Autodesk Inventor part; units mm, degrees
ref_plane "YZ Plane" through (0, 0, 0) normal (1, 0, 0) x (0, 1, 0)
ref_plane "XZ Plane" through (0, 0, 0) normal (0, 1, 0) x (-1, 0, 0)
ref_plane "XY Plane" through (0, 0, 0) normal (0, 0, 1) x (1, 0, 0)
sketch "Sketch1" plane through (0, 0, 0) normal (1, 0, 0) x (0, 1, 0)
  line L0 (-219.6367, 33.4515) -> (-197.6397, 20.7515)
  line L1 (-197.6397, 20.7515) -> (-184.9397, 42.7485)
  line L2 (-184.9397, 42.7485) -> (-206.9367, 55.4485)
  line L3 (-206.9367, 55.4485) -> (-219.6367, 33.4515)
  line L4 (-219.6367, 33.4515) -> (-184.9397, 42.7485) construction
  line L5 (-197.6397, 20.7515) -> (-206.9367, 55.4485) construction
  circle A0 centre (-38.1, 41.275) radius 38.1
  line L6 (0, 0) -> (-228.6, 0)
  line L7 (-228.6, 0) -> (-228.6, -25.4)
  line L8 (-228.6, -25.4) -> (0, -25.4)
  line L9 (0, -25.4) -> (0, 0)
  line L10 (0, 0) -> (-228.6, -25.4) construction
  line L11 (-228.6, 0) -> (0, -25.4) construction
  line L12 (-38.1, 3.175) -> (-132.0434, 3.175)
  arc A1 (-197.6397, 20.7515) -> (-132.0434, 3.175) centre (-132.0434, 134.3676) ccw
  circle A2 centre (-38.1, 41.275) radius 44.45
  arc A3 (-184.9397, 42.7485) -> (-79.7897, 25.8552) centre (-110.2136, 172.1778) ccw
  circle A4 centre (-101.6, 41.275) radius 7.3323
  line L13 (-107.95, 44.9412) -> (-101.6, 48.6073)
  line L14 (-101.6, 48.6073) -> (-95.25, 44.9412)
  line L15 (-95.25, 44.9412) -> (-95.25, 37.6088)
  line L16 (-95.25, 37.6088) -> (-101.6, 33.9427)
  line L17 (-101.6, 33.9427) -> (-107.95, 37.6088)
  line L18 (-107.95, 37.6088) -> (-107.95, 44.9412)
  point P0 (-202.2882, 38.1)
  point P1 (-114.3, -12.7)
  point P2 (-60.9953, 3.175)
  dimension "d0" = 76.2
  dimension "d1" = 25.4
  dimension "d2" = 60
  dimension "d3" = 41.275
  dimension "d4" = 38.1
  dimension "d5" = 146.847
  dimension "d6" = 20.7515
  dimension "d7" = 228.6
  dimension "d8" = 88.9
  dimension "d23" = 12.7
  dimension "d24" = 63.5
extrude "Extrusion1" add sketch "Sketch1" along normal mid plane 177.8 contours L1 A3 A2 L12 A1
sketch "Sketch2" plane through (-88.9, -197.6397, 20.7515) normal (0, -0.866, 0.5) x (1, 0, 0)
  line L0 (0, 0) -> (177.8, 0)
  line L1 (177.8, 25.4) -> (177.8, 0)
  point P0 (88.9, 80.8485)
  point P1 (152.4, 12.7)
  dimension "d11" = 12.7
  dimension "d12" = 25.4
hole "Hole1" at (63.5, -191.2897, 31.75) direction (0, 0.866, -0.5) diameter 4.445 depth 38.1 counterbore diameter 5.588 counterbore depth 8.255
pattern_linear "Rectangular Pattern1" count 6 spacing 25.4 along (-1, 0, 0) of "Hole1"
properties part number "FlyWheel Alligner"
Part model, mm, in its own coordinate system. A direction names the side the tool comes from. Give positions to 0.01 mm unless a question says otherwise; leave off trailing zeros. Write each loop counter-clockwise with the first axis right and the second up, starting at its lowest first coordinate (ties: lowest second). Pieces come first, ordered by that corner, then holes. Notation, with made-up numbers: (77.25, -20) -> (128.25, -20) arc R22 ccw to (128.25, 14) -> close; hole circle Ø11 at (-18.75, 79). An arc over 180 degrees is marked (long way). Put each result on its own line as item: value. Start each with the question number.
Item 1: Which spindle directions (+Z, -Z, +X, -X, +Y, -Y) get a long thin tool onto all of the face, cutting with end or side? Do faces 4 (the face through (-1.24, -133.17, 24.5)), 5 (the face through (-38.131, -158.279, 12.727)). Say none if no direction does.
Item 2: Cut at B-B (y = -113.5). List the corners of the cut face in (x, z) (3 decimals), then the cut area to 3 significant figures.
Item 3: Pull direction X, two halves, no side cores. Call faces 1 (the face through (-35.62, -188.31, 28.54)), 2 (the face through (-1, -96, 3.175)), 3 (the face through (-88.9, -130, 19)): pulls with the +X half, pulls with the -X half, needs draft (parallel to the pull), parting line crosses it, or undercut.
Item 4: Cut at C-C (z = 36.5). List the corners of the cut face in (x, y), then the cut area to 3 significant figures.
Item 5: Pin check, flat tips, straight feed: pin 1 Ø1 at (x, y) = (-45.5, -163.5) entering from +Z; pin 2 Ø1 at (x, z) = (-23.5, 17) entering from -Y; pin 3 Ø5 at (x, y) = (22.5, -166) entering from -Z. Stop position of each tip, or through.
Item 6: Wall check: L1, parallel to Z at x = 41.5, y = -80 (3 decimals); L2, parallel to Y at x = 62, z = 22; L3, parallel to Z at x = 19, y = -108 (3 decimals). Give the ranges that are in metal, low to high. Write a range as [from, to].
Answer list:
1. face 4: +Z, +X, -X
1. face 5: none
2. outline: (-88.9, 3.175) -> (88.9, 3.175) -> (88.9, 22.762) -> (-88.9, 22.762) -> close
2. area: 3,480 mm2
3. face 1: undercut
3. face 2: needs draft
3. face 3: pulls with the -X half
4. outline: (-88.9, -188.55) -> (88.9, -188.55) -> (88.9, -172.88) -> (-88.9, -172.88) -> close
4. area: 2,790 mm2
5. pin 1: stops at z = 32.74
5. pin 2: stops at y = -191.65
5. pin 3: stops at z = 7
6. L1: z = [3.175, 25.812]
6. L2: y = [-196.92, -177.68], [-171.12, -78.15]
6. L3: z = [3.175, 22.742]
